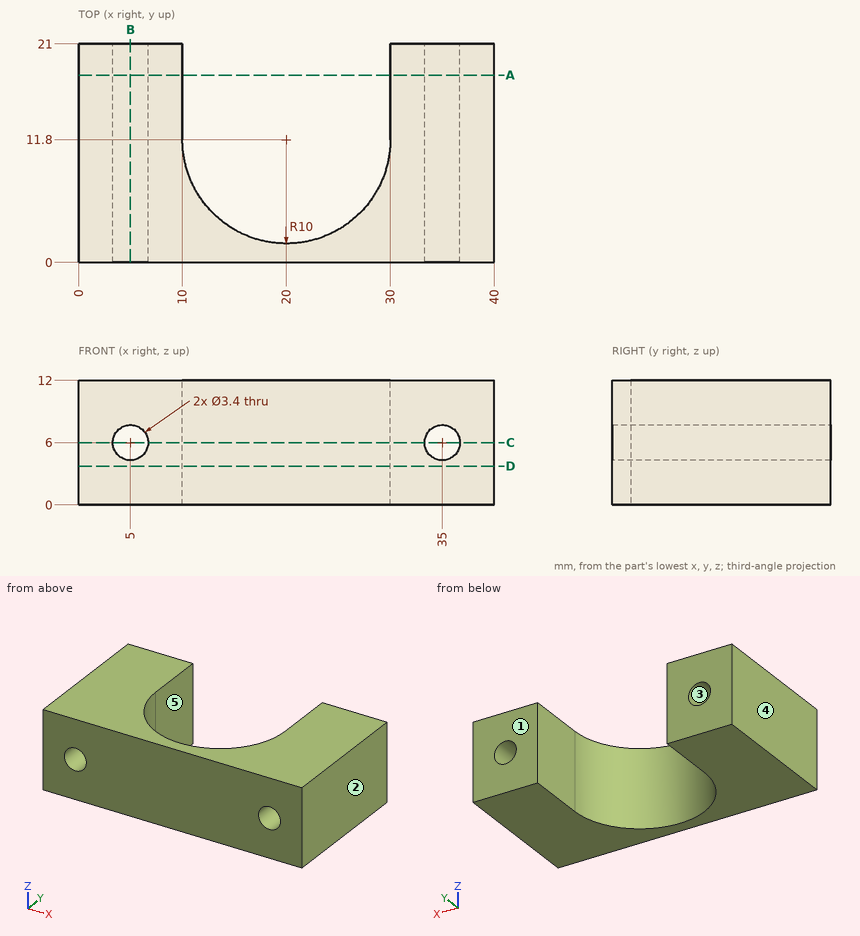
The figure shows three views and two pictorial views of one solid part (mm, origin at its lowest corner). Answer the questions. A direction names the side the tool comes from. Coordinates: 2 decimals unless noted, no trailing zeros. Order: outer loops, then holes, each group sorted by start corner. A loop starts at its lowest first (then second) coordinate and runs counter-clockwise, first axis right, second up. Notation, with made-up numbers: (37, 62.5) - (76, 62.5) arc R25 ccw to (76, 89.5) - close; hole circle Ø6 at (61, -4.75). An arc over 180 degrees is marked (long way). Answer as a JSON object with one key per item and string values.
1. A tool of negligible diameter and unlimited length cuts with its end or side. For the marked faces 4 and 5, from which of +Z, -Z, +X, -X, +Y, -Y can it reach the whole face along a straight path? Write none if from no direction.
Output values:
{"face 4": "+Z, -Z, -X, +Y, -Y", "face 5": "+Z, -Z, +Y"}
2. Find section A-A on y = 18. Determine the outline of the cut face in (x, z).
Output values:
{"outline": "(0, 0) - (10, 0) - (10, 12) - (0, 12) - close; (30, 0) - (40, 0) - (40, 12) - (30, 12) - close; hole circle Ø3.4 at (5, 6); hole circle Ø3.4 at (35, 6)"}
3. Find section C-C on z = 6. Determine the outline of the cut face in (x, y), plus the area to 3 significant figures.
Output values:
{"outline": "(0, 0) - (3.3, 0) - (3.3, 21) - (0, 21) - close; (6.7, 0) - (33.3, 0) - (33.3, 21) - (30, 21) - (30, 11.8) arc R10 cw to (10, 11.8) - (10, 21) - (6.7, 21) - close; (36.7, 0) - (40, 0) - (40, 21) - (36.7, 21) - close", "area": "356 mm²"}
4. Consider line 1 (X direction, y = 15, z = 6); line 2 (Z direction, x = 35, y = 15); line 3 (X direction, y = 13, z = 2.75). Determine where each line is inside the solid, lowest interval first.
Output values:
{"line 1": "x = 0 to 3.3, 6.7 to 10, 30 to 33.3, 36.7 to 40", "line 2": "z = 0 to 4.3, 7.7 to 12", "line 3": "x = 0 to 10, 30 to 40"}
5. Find section D-D on z = 3.75. Determine the outline of the cut face in (x, y), plus the area to 3 significant figures.
Output values:
{"outline": "(0, 0) - (40, 0) - (40, 21) - (30, 21) - (30, 11.8) arc R10 cw to (10, 11.8) - (10, 21) - (0, 21) - close", "area": "499 mm²"}
6. Each of these flat-tipped pins is pushed along its axis until it touches: P1, Ø2, axis at x = 35, z = 6, coming from the -Y side; P2, Ø5, axis at x = 14.5, z = 7, coming from the +Y side; P3, Ø5, axis at x = 23, z = 3.5, coming from the -Y side. Where does it stop, or does it pass through?
Output values:
{"P1": "passes through", "P2": "stops at y = 5.8", "P3": "stops at y = 0"}
7. The mould has two halves that part along X. Classify the marked faces 1, 2 and 3: +X half, -X half, draft (parallel to the pull), parting line (faces both ways), or undercut.
Output values:
{"face 1": "draft", "face 2": "+X half", "face 3": "undercut"}
8. Find section B-B on x = 5. Determine the outline of the cut face in (y, z).
Output values:
{"outline": "(0, 0) - (21, 0) - (21, 4.3) - (0, 4.3) - close; (0, 7.7) - (21, 7.7) - (21, 12) - (0, 12) - close"}
